CAD build for the part. Positions are in the model's coordinates, mm. Face numbers are marked on the shaded views. A direction names the side the tool comes from. Round coordinates to 2 decimals unless told otherwise and drop trailing zeros. Loops run counter-clockwise (first coordinate to the right, second up) from the corner with the lowest first, then second, coordinate; pieces in that order, holes last. Notation, with made-up numbers: M 71.5,-12 L 111.5,-12 A22 cw 111.5,3 Z; hole C -22,-23.75 d9. An arc over 180 degrees is marked long. One line per item, written item: value. Start each with the question number.
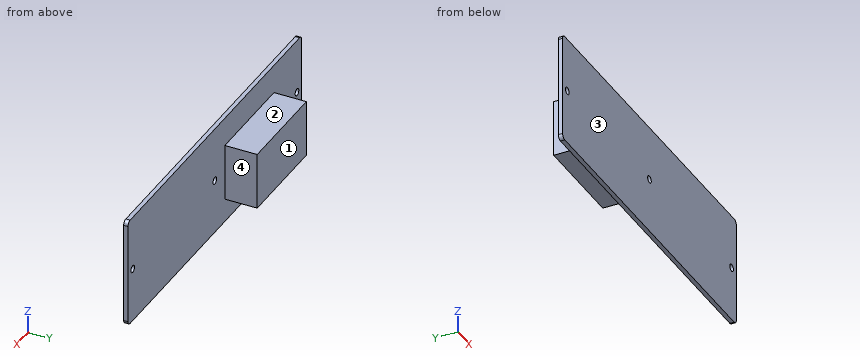
from build123d import *

# Parameters (mm, degrees)
SKETCH1_W           = 158
SKETCH1_H           = 51
BOSS_EXTRUDE1_DEPTH = 2
SKETCH2_R           = 1.65
CUT_EXTRUDE1_DEPTH  = 3
FILLET1_R           = 2
SKETCH3_W           = 44.679431241
SKETCH3_H           = 26.501035196
BOSS_EXTRUDE2_DEPTH = 15


with BuildPart() as part:
    # Sketch1 → Boss-Extrude1 (new body)
    with BuildSketch(Plane(origin=(0, 0, 0), x_dir=(1, 0, 0), z_dir=(0, 1, 0))):
        with Locations((79, 25.5)):
            Rectangle(SKETCH1_W, SKETCH1_H)
    extrude(amount=BOSS_EXTRUDE1_DEPTH)

    # Sketch2 → Cut-Extrude1 (cut, through all)
    with BuildSketch(Plane(origin=(0, 2, 0), x_dir=(1, 0, 0), z_dir=(0, 1, 0))):
        with Locations((4.3, 25.5)):
            Circle(SKETCH2_R)
        with Locations((153.7, 25.5)):
            Circle(SKETCH2_R)
        with Locations((79, 25.5)):
            Circle(SKETCH2_R)
    extrude(amount=-CUT_EXTRUDE1_DEPTH, mode=Mode.SUBTRACT)

    # Fillet1
    fillet1_edges = [part.edges().sort_by_distance(p)[0] for p in [
        (0, 1, -51),
        (158, 1, -51),
        (158, 1, 0),
        (0, 1, 0),
    ]]
    fillet(fillet1_edges, radius=FILLET1_R)

    # Sketch3 → Boss-Extrude2 (add)
    with BuildSketch(Plane(origin=(0, 2, 0), x_dir=(1, 0, 0), z_dir=(0, 1, 0))):
        with Locations((47.571086358, 26.704592509)):
            Rectangle(SKETCH3_W, SKETCH3_H)
    extrude(amount=BOSS_EXTRUDE2_DEPTH)


solid = part.part
(1) Flat gauge pins, fed straight in: P1, Ø5.5, axis at x = 153.7, z = -25.5, coming from the -Y side; P2, Ø3, axis at x = 96, y = 4, coming from the -Z side; P3, Ø2, axis at y = 5.5, z = -28, coming from the +X side; P4, Ø4.5, axis at y = 6.5, z = -31, coming from the -X side. Where does each tip first touch, or does it go through?
(2) Slice it at C-C, the plane z = -18. List the corners of the cut face in (x, y).
(3) Probe L1, parallel to X at y = 0.85, z = -25.5; L2, parallel to Z at x = 79, y = 1.5; L3, parallel to X at y = 2.5, z = -27.5. List the from-to ranges inside material, lowest first.
(4) Slice it at B-B, the plane x = 153.7. List the corners of the cut face in (y, z), and give its area (3 significant figures).
(5) Slice it at D-D, the plane x = 67. List the corners of the cut face in (y, z), and give its area (3 significant figures).
(6) Mould opens along X. For the marked faces 3 and 4 say: pulls with the +X half, pulls with the -X half, needs draft (parallel to the pull), parting line crosses it, or undercut.
(7) Which spindle directions (+Z, -Z, +X, -X, +Y, -Y) get a long thin tool onto all of the face, cutting with end or side? Do the marked faces 1 and 2. Say none if no direction does.
(8) Slice it at A-A, the plane z = -25.5. List the corners of the cut face in (x, y), and give its area (3 significant figures).
Check result:
1. P1: stops at y = 0
1. P2: passes through
1. P3: stops at x = 69.91
1. P4: stops at x = 25.23
2. outline: M 0,0 L 158,0 L 158,2 L 69.91,2 L 69.91,17 L 25.23,17 L 25.23,2 L 0,2 Z
3. L1: x = 0 to 2.65, 5.95 to 77.35, 80.65 to 152.05, 155.35 to 158
3. L2: z = -51 to -27.15, -23.85 to 0
3. L3: x = 25.23 to 69.91
4. outline: M 0,-51 L 2,-51 L 2,-27.15 L 0,-27.15 Z; M 0,-23.85 L 2,-23.85 L 2,0 L 0,0 Z
4. area: 95.4 mm^2
5. outline: M 0,-51 L 2,-51 L 2,-39.96 L 17,-39.96 L 17,-13.45 L 2,-13.45 L 2,0 L 0,0 Z
5. area: 500 mm^2
6. face 3: needs draft
6. face 4: pulls with the +X half
7. face 1: +Z, -Z, +X, -X, +Y
7. face 2: +Z, +X, -X, +Y
8. outline: M 0,0 L 2.65,0 L 2.65,2 L 0,2 Z; M 5.95,0 L 77.35,0 L 77.35,2 L 69.91,2 L 69.91,17 L 25.23,17 L 25.23,2 L 5.95,2 Z; M 80.65,0 L 152.05,0 L 152.05,2 L 80.65,2 Z; M 155.35,0 L 158,0 L 158,2 L 155.35,2 Z
8. area: 966 mm^2
